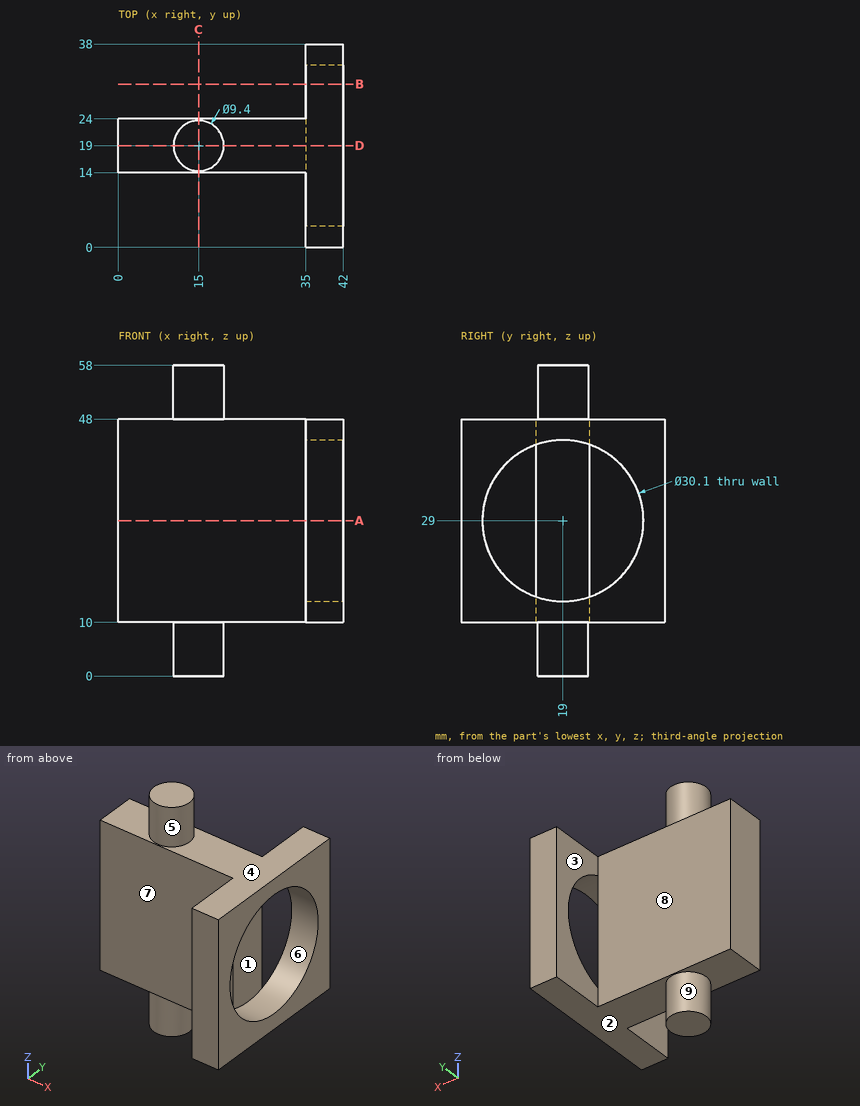
Geometry: see drawing. Coordinates: mm, zero at the bounding-box minimum. A direction names the side the tool comes from. Coordinates: 2 decimals unless noted, no trailing zeros. Order: outer loops, then holes, each group sorted by start corner. A loop starts at its lowest first (then second) coordinate and runs counter-clockwise, first axis right, second up. Notation, with made-up numbers: (77, 52.25) - (89, 52.25) arc R17 ccw to (89, 58.25) - close; hole circle Ø5 at (-19, -15.75). An arc over 180 degrees is marked (long way). Write each question's results on one line, items separated by ' | '.
1) Section D-D, the plane y = 19. Return loops of the section in (x, z).
Results list:
outline: (0, 10) - (10.3, 10) - (10.3, 0) - (19.7, 0) - (19.7, 10) - (42, 10) - (42, 13.95) - (35, 13.95) - (35, 44.05) - (42, 44.05) - (42, 48) - (19.7, 48) - (19.7, 58) - (10.3, 58) - (10.3, 48) - (0, 48) - close
2) Pull-direction query (Z, two-part tool) for the marked faces 1, 2, 3 and 4; classes: pulls with the +Z half, pulls with the -Z half, needs draft (parallel to the pull), parting line crosses it, or undercut.
Results list:
face 1: undercut | face 2: pulls with the -Z half | face 3: needs draft | face 4: pulls with the +Z half
3) Section B-B, the plane y = 30.5. Return loops of the section in (x, z), plus the area to 3 significant figures.
Results list:
outline: (35, 10) - (42, 10) - (42, 19.29) - (35, 19.29) - close; (35, 38.71) - (42, 38.71) - (42, 48) - (35, 48) - close | area: 130 mm^2
4) Pin query (flat end, axial travel): pin 1 (10.5 mm diameter, centred on x = 25.5, z = 27.5, fed in from +Y); pin 2 (7 mm diameter, centred on y = 4.5, z = 22.5, fed in from -X); pin 3 (17.5 mm diameter, centred on x = 18, z = 30, fed in from -Y); pin 4 (5 mm diameter, centred on x = 18.5, y = 22, fed in from -Z). Return the tip coordinate at first contact, or that it passes through.
Results list:
pin 1: y = 24 | pin 2: x = 35 | pin 3: y = 14 | pin 4: z = 0
5) Section C-C, the plane x = 15. Return loops of the section in (y, z).
Results list:
outline: (14, 10) - (14.3, 10) - (14.3, 0) - (23.7, 0) - (23.7, 10) - (24, 10) - (24, 48) - (23.7, 48) - (23.7, 58) - (14.3, 58) - (14.3, 48) - (14, 48) - close
6) Section A-A, the plane z = 29. Return loops of the section in (x, y), plus the area to 3 significant figures.
Results list:
outline: (0, 14) - (35, 14) - (35, 24) - (0, 24) - close; (35, 0) - (42, 0) - (42, 3.95) - (35, 3.95) - close; (35, 34.05) - (42, 34.05) - (42, 38) - (35, 38) - close | area: 405 mm^2
7) Line query: line 1 (Y direction, x = 39.5, z = 29); line 2 (Z direction, x = 39, y = 19); line 3 (Y direction, x = 23, z = 47). Output: solid intervals per line, ascending. Write a range as from..to.
Results list:
line 1: 0..3.95, 34.05..38 | line 2: 10..13.95, 44.05..48 | line 3: 14..24
8) Set-up query: the marked faces 5, 6, 7, 8 and 9. Return all of +Z, -Z, +X, -X, +Y, -Y with unobstructed straight access to the full face (end or side cutting, diameter ignored); none if empty.
Results list:
face 5: +Z | face 6: +X | face 7: +Z, -Z, -X, -Y | face 8: +Z, -Z, -X, +Y | face 9: -Z
